Part model, mm, in its own coordinate system. A direction names the side the tool comes from. Round coordinates to 2 decimals unless told otherwise and drop trailing zeros. Loops run counter-clockwise (first coordinate to the right, second up) from the corner with the lowest first, then second, coordinate; pieces in that order, holes last.
(1) Cut at B-B on z = 95.5. List the corners of the cut face in (x, y).
(2) Probe probe 1 along X at (y, z) = (-23, 131); probe 2 along Y at (x, z) = (41, 18); probe 3 along X at (y, z) = (45, 125). List the from-to ranges inside material, lowest first.
(3) Cut at A-A on y = -24. List the corners of the cut face in (x, z).
(4) Cut at D-D on z = 117. List the corners of the cut face in (x, y), then the cut area to 3 significant figures.
(5) Tool access for faces 1 (the face through (-24, -31.171, 10)), 2 (the face through (82, -6.171, 6)), 3 (the face through (82, 25.829, 9)), 4 (the face through (11.152, -32, 95)): list every direction of +Z, -Z, +X, -X, +Y, -Y with a clear straight run to the whole face (end or side of a thin tool).
(6) Cut at C-C on x = -15. List the corners of the cut face in (y, z).
(7) Mould opens along Y. For faces 5 (the face through (-26, -34, 15)), 6 (the face through (1, -16.171, 95)), 7 (the face through (79.128, 0.697, 2.465)) say: +Y half, -Y half, draft (parallel to the pull), parting line (faces both ways), or undercut.
(8) Flat gauge pins, fed straight in: pin 1 (12.5 mm diameter, centred on x = -2, z = 133.5, fed in from -Y); pin 2 (0.6 mm diameter, centred on y = -27, z = 94.5, fed in from -X); pin 3 (6 mm diameter, centred on x = 5.5, z = 132, fed in from +Y); pin 4 (3 mm diameter, centred on x = -24.35, z = 15, fed in from +Y). Where does each tip first touch, or does it go through?
from build123d import *

# Parameters (mm, degrees)
SKETCH_1_W           = 120
SKETCH_1_H           = 95
EXTRUDE_1_DEPTH      = 150
SKETCH_2_W           = 115
SKETCH_2_H           = 85
CUT_EXTRUDE_1_DEPTH  = 150
CUT_EXTRUDE_2_DEPTH  = 150
SKETCH_5_W           = 10
SKETCH_5_H           = 35
SKETCH_5_R           = 1.65
EXTRUDE_2_DEPTH      = 5
EXTRUDE_START        = -33
EXTRUDE_3_DEPTH      = 3
EXTRUDE_START_2      = 52
EXTRUDE_4_DEPTH      = 3
SKETCH_8_W           = 10
SKETCH_8_H           = 20
SKETCH_8_R           = 1.65
CUT_EXTRUDE_3_DEPTH  = 5
SKETCH_10_R          = 1.65
CUT_EXTRUDE_4_DEPTH  = 195.788985905
SKETCH_22_R          = 7.75
CUT_EXTRUDE_8_DEPTH  = 199.407311022
SKETCH_24_R          = 9.75
SKETCH_24_R_2        = 7.75
EXTRUDE_7_DEPTH      = 15
SKETCH_26_R          = 9.75
EXTRUDE_8_DEPTH      = 5
SKETCH_31_W          = 40.5
SKETCH_31_H          = 21
CUT_EXTRUDE_11_DEPTH = 8
SKETCH_32_W          = 5
SKETCH_32_H          = 14
CUT_EXTRUDE_12_DEPTH = 200.355835204
SKETCH_33_W          = 55
SKETCH_33_H          = 55
CUT_EXTRUDE_13_DEPTH = 1
EXTRUDE_9_DEPTH      = 5


with BuildPart() as part:
    # 草图1 → 凸台-拉伸1 (new body)
    with BuildSketch(Plane.XY):
        with Locations((30.651801029, 11.329331046)):
            Rectangle(SKETCH_1_W, SKETCH_1_H)
    extrude(amount=EXTRUDE_1_DEPTH)

    # 草图2 → 切除-拉伸1 (cut)
    with BuildSketch(Plane.XY.offset(150)):
        with Locations((28.151801029, 16.329331046)):
            Rectangle(SKETCH_2_W, SKETCH_2_H)
    extrude(amount=-CUT_EXTRUDE_1_DEPTH, mode=Mode.SUBTRACT)

    # 草图3 → 切除-拉伸2 (cut)
    with BuildSketch(Plane(origin=(90.651801029, 0, 0), x_dir=(0, 0, -1), z_dir=(1, 0, 0))):
        Polygon((-150, 58.829331046), (-150, -26.170668954), (0, 58.829331046), align=None)
    extrude(amount=-CUT_EXTRUDE_2_DEPTH, mode=Mode.SUBTRACT)

    # 草图5 → 凸台-拉伸2 (add)
    with BuildSketch(Plane(origin=(0, 0, 0), x_dir=(-1, 0, 0), z_dir=(0, 0, -1))):
        with Locations((-80.651801029, 11.329331046)):
            Rectangle(SKETCH_5_W, SKETCH_5_H)
        with Locations((-80.651801029, 21.329331046)):
            Circle(SKETCH_5_R, mode=Mode.SUBTRACT)
        with Locations((-80.651801337, 11.329331046)):
            Circle(SKETCH_5_R, mode=Mode.SUBTRACT)
        with Locations((-80.651801337, 1.329331046)):
            Circle(SKETCH_5_R, mode=Mode.SUBTRACT)
    extrude(amount=-EXTRUDE_2_DEPTH)

    # 草图6 → 凸台-拉伸3 (add)
    with BuildSketch(Plane(origin=(0, -36.170668954, 0), x_dir=(-1, 0, 0), z_dir=(0, -1, 0)).offset(EXTRUDE_START)):
        Polygon((-85.651801029, -5), (-75.651801029, -5), (-85.651801029, -15), align=None)
    extrude(amount=EXTRUDE_3_DEPTH)

    # 草图7 → 凸台-拉伸4 (add)
    with BuildSketch(Plane(origin=(0, -26.170668954, 0), x_dir=(1, 0, 0), z_dir=(0, 1, 0)).offset(EXTRUDE_START_2)):
        Polygon((75.651801029, -5), (85.651801029, -5), (85.651801029, -15), align=None)
    extrude(amount=EXTRUDE_4_DEPTH)

    # 草图8 → 切除-拉伸3 (cut)
    with BuildSketch(Plane(origin=(0, -26.170668954, 0), x_dir=(1, 0, 0), z_dir=(0, 1, 0))):
        with Locations((-24.348198971, -10)):
            Rectangle(SKETCH_8_W, SKETCH_8_H)
        with Locations(Location((-24.348198971, -5, 0), (0, 0, 180))):
            Circle(SKETCH_8_R, mode=Mode.SUBTRACT)
        with Locations(Location((-24.348198971, -15, 0), (0, 0, 180))):
            Circle(SKETCH_8_R, mode=Mode.SUBTRACT)
    extrude(amount=-CUT_EXTRUDE_3_DEPTH, mode=Mode.SUBTRACT)

    # 草图10 → 切除-拉伸4 (cut, through all)
    with BuildSketch(Plane(origin=(0, -26.170668954, 0), x_dir=(1, 0, 0), z_dir=(0, 1, 0))):
        with Locations(Location((-24.348198971, -5, 0), (0, 0, 180))):
            Circle(SKETCH_10_R)
        with Locations(Location((-24.348198971, -15, 0), (0, 0, 180))):
            Circle(SKETCH_10_R)
    extrude(amount=-CUT_EXTRUDE_4_DEPTH, mode=Mode.SUBTRACT)

    # 草图22 → 切除-拉伸8 (cut, through all)
    with BuildSketch(Plane(origin=(76.451044211, -36.170668954, 11.627382734), x_dir=(-1, 0, 0), z_dir=(0, -1, 0))):
        with Locations(Location((75.799243182, -83.872617266, 0), (0, 0, 90))):
            Circle(SKETCH_22_R)
        with Locations(Location((75.799243182, -119.872617266, 0), (0, 0, 90))):
            Circle(SKETCH_22_R)
    extrude(amount=-CUT_EXTRUDE_8_DEPTH, mode=Mode.SUBTRACT)

    # 草图24 → 凸台-拉伸7 (add)
    # profile 1 of 2: a face of its own
    with BuildSketch(Plane(origin=(76.451044211, -36.170668954, 11.627382734), x_dir=(-1, 0, 0), z_dir=(0, -1, 0))):
        with Locations(Location((75.799243182, -83.872617266, 0), (0, 0, 90))):
            Circle(SKETCH_24_R)
        with Locations(Location((75.799243182, -83.872617266, 0), (0, 0, 90))):
            Circle(SKETCH_24_R_2, mode=Mode.SUBTRACT)
    # profile 2 of 2: a face of its own
    with BuildSketch(Plane(origin=(76.451044211, -36.170668954, 11.627382734), x_dir=(-1, 0, 0), z_dir=(0, -1, 0))):
        with Locations(Location((75.799243182, -119.872617266, 0), (0, 0, 90))):
            Circle(SKETCH_24_R)
        with Locations(Location((75.799243182, -119.872617266, 0), (0, 0, 90))):
            Circle(SKETCH_24_R_2, mode=Mode.SUBTRACT)
    extrude(amount=-EXTRUDE_7_DEPTH)

    # 草图26 → 凸台-拉伸8 (add)
    with BuildSketch(Plane(origin=(-76.451044211, -21.170668954, 11.627382734), x_dir=(1, 0, 0), z_dir=(0, 1, 0))):
        with Locations((77.10284524, -83.872617266)):
            Circle(SKETCH_26_R)
        with Locations((77.10284524, -119.872617266)):
            Circle(SKETCH_26_R)
    extrude(amount=EXTRUDE_8_DEPTH)

    # 草图31 → 切除-拉伸11 (cut)
    with BuildSketch(Plane.XZ.offset(36.170668954)):
        with Locations((-9.098198971, 131.5)):
            Rectangle(SKETCH_31_W, SKETCH_31_H)
        with Locations((-9.098198971, 95.5)):
            Rectangle(SKETCH_31_W, SKETCH_31_H)
    extrude(amount=-CUT_EXTRUDE_11_DEPTH, mode=Mode.SUBTRACT)

    # 草图32 → 切除-拉伸12 (cut, through all)
    with BuildSketch(Plane.XZ.offset(36.170668954)):
        with Locations((-26.848198971, 130)):
            Rectangle(SKETCH_32_W, SKETCH_32_H)
        with Locations((-26.848198971, 94)):
            Rectangle(SKETCH_32_W, SKETCH_32_H)
    extrude(amount=-CUT_EXTRUDE_12_DEPTH, mode=Mode.SUBTRACT)

    # 草图33 → 切除-拉伸13 (cut)
    with BuildSketch(Plane.XZ.offset(36.170668954)):
        with Locations((58.151801029, 117.5)):
            Rectangle(SKETCH_33_W, SKETCH_33_H)
    extrude(amount=-CUT_EXTRUDE_13_DEPTH, mode=Mode.SUBTRACT)

    # 草图34 → 凸台-拉伸9 (add)
    with BuildSketch(Plane(origin=(90.651801029, 0, 0), x_dir=(0, 0, -1), z_dir=(1, 0, 0))):
        with BuildLine():
            Line((-150, -26.170668954), (-150, 28.829331046))
            ThreePointArc((-150, 28.829331046), (-141.213203436, 50.042534482), (-120, 58.829331046))
            Line((-120, 58.829331046), (0, 58.829331046))
            Line((0, 58.829331046), (-150, -26.170668954))
        make_face()
    extrude(amount=-EXTRUDE_9_DEPTH)


solid = part.part
Final values:
1. outline: (-24.35, -28.17) - (-7.1, -28.17) - (-7.1, -21.17) - (8.4, -21.17) - (8.4, -28.17) - (11.15, -28.17) - (11.15, -36.17) - (30.65, -36.17) - (30.65, -35.17) - (85.65, -35.17) - (85.65, -36.17) - (90.65, -36.17) - (90.65, 58.83) - (85.65, 58.83) - (85.65, -26.17) - (10.4, -26.17) - (10.4, -16.17) - (-9.1, -16.17) - (-9.1, -26.17) - (-24.35, -26.17) - close
2. probe 1: x = -9.09 to -7.08, 8.39 to 10.39, 85.65 to 90.65
2. probe 2: y = -36.17 to -26.17
2. probe 3: x = 85.65 to 90.65
3. outline: circle Ø19.5 at (0.65, 95.5); circle Ø19.5 at (0.65, 131.5); (85.65, 0) - (90.65, 0) - (90.65, 150) - (85.65, 150) - close; hole circle Ø15.5 at (0.65, 95.5); hole circle Ø15.5 at (0.65, 131.5)
4. outline: (-29.35, -36.17) - (30.65, -36.17) - (30.65, -35.17) - (85.65, -35.17) - (85.65, -36.17) - (90.65, -36.17) - (90.65, 58.83) - (85.65, 58.83) - (85.65, -26.17) - (-29.35, -26.17) - close
4. area: 1,570 mm2
5. face 1: -Z, -X, +Y
5. face 2: +Z, -Z, -X
5. face 3: +Z, -X
5. face 4: -X, -Y
6. outline: (-36.17, 0) - (-26.17, 0) - (-26.17, 150) - (-36.17, 150) - (-36.17, 142) - (-28.17, 142) - (-28.17, 121) - (-36.17, 121) - (-36.17, 106) - (-28.17, 106) - (-28.17, 85) - (-36.17, 85) - close
7. face 5: draft
7. face 6: +Y half
7. face 7: undercut
8. pin 1: stops at y = -28.17
8. pin 2: stops at x = -24.35
8. pin 3: stops at y = -16.17
8. pin 4: passes through
